Answer from the drawing. Dimensions are ordinates in mm from the lowest x, y and z of the part. A direction names the side the tool comes from. Coordinates: 2 decimals unless noted, no trailing zeros. Write each loop counter-clockwise with the first axis right and the second up, starting at its lowest first coordinate (ties: lowest second). Pieces come first, ordered by that corner, then holes. Notation, with made-up numbers: (11.5, 85.5) -> (37.5, 85.5) arc R20 ccw to (37.5, 106.5) -> close; hole circle Ø8 at (-27, -13). An arc over 180 degrees is marked (long way). Use CSV: the item, a comma, the result in double quotes.
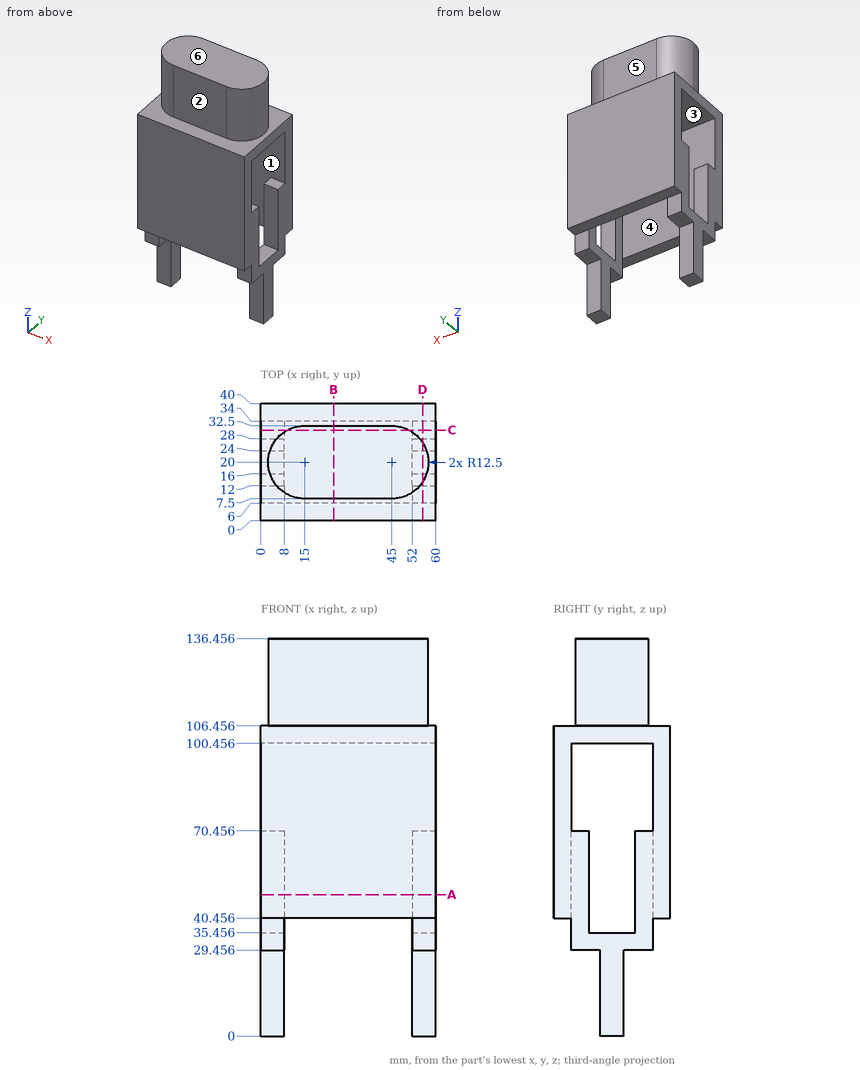
1. For a pull along Z with two mould halves and no side action, classify the marked faces 4, 5 and 6 as pulls with the +Z half, pulls with the -Z half, needs draft (parallel to the pull), parting line crosses it, or undercut.
Solutions:
face 4,"undercut"
face 5,"needs draft"
face 6,"pulls with the +Z half"
2. A cutting plane is placed at B-B (x = 25). Give the vertices of the cut face in (y, z).
Solutions:
outline,"(0, 40.46) -> (6, 40.46) -> (6, 100.46) -> (34, 100.46) -> (34, 40.46) -> (40, 40.46) -> (40, 106.46) -> (32.5, 106.46) -> (32.5, 136.46) -> (7.5, 136.46) -> (7.5, 106.46) -> (0, 106.46) -> close"
3. A cutting plane is placed at A-A (z = 48.5). Give the vertices of the cut face in (x, y).
Solutions:
outline,"(0, 0) -> (60, 0) -> (60, 12) -> (52, 12) -> (52, 6) -> (8, 6) -> (8, 12) -> (0, 12) -> close; (0, 28) -> (8, 28) -> (8, 34) -> (52, 34) -> (52, 28) -> (60, 28) -> (60, 40) -> (0, 40) -> close"
4. Find the intervals of material crossed by line 1 along Y through (x, z) = (25, 81); line 2 along X through (y, z) = (20, 9.5); line 3 along Z through (x, y) = (56.5, 18.5), in increasing order.
Solutions:
line 1,"y = 0 to 6, 34 to 40"
line 2,"x = 0 to 8, 52 to 60"
line 3,"z = 0 to 35.46, 100.46 to 136.46"
5. Each of these flat-tipped pins is pushed along its axis until it touches: pin 1 Ø9 at (x, z) = (54.5, 14) entering from +Y; pin 2 Ø2.5 at (x, z) = (4, 33.5) entering from +Y; pin 3 Ø9 at (x, y) = (5, 29) entering from -Z. Where does it stop, or does it pass through?
Solutions:
pin 1,"stops at y = 24"
pin 2,"stops at y = 34"
pin 3,"stops at z = 29.46"
6. A cutting plane is placed at C-C (y = 31). Give the vertices of the cut face in (x, z), and give its area (3 significant figures).
Solutions:
outline,"(0, 29.46) -> (8, 29.46) -> (8, 70.46) -> (0, 70.46) -> close; (0, 100.46) -> (60, 100.46) -> (60, 106.46) -> (50.94, 106.46) -> (50.94, 136.46) -> (9.06, 136.46) -> (9.06, 106.46) -> (0, 106.46) -> close; (52, 29.46) -> (60, 29.46) -> (60, 70.46) -> (52, 70.46) -> close"
area,"2,270 mm^2"
7. A cutting plane is placed at D-D (x = 55.5). Give the vertices of the cut face in (y, z).
Solutions:
outline,"(0, 40.46) -> (6, 40.46) -> (6, 29.46) -> (16, 29.46) -> (16, 0) -> (24, 0) -> (24, 29.46) -> (34, 29.46) -> (34, 40.46) -> (40, 40.46) -> (40, 106.46) -> (26.78, 106.46) -> (26.78, 136.46) -> (13.22, 136.46) -> (13.22, 106.46) -> (0, 106.46) -> close; hole (6, 70.46) -> (12, 70.46) -> (12, 35.46) -> (28, 35.46) -> (28, 70.46) -> (34, 70.46) -> (34, 100.46) -> (6, 100.46) -> close"
8. A tool of negligible diameter and unlimited length cuts with its end or side. For the marked faces 1, 2 and 3, from which of +Z, -Z, +X, -X, +Y, -Y can it reach the whole face along a straight path? Write none if from no direction.
Solutions:
face 1,"none"
face 2,"+Z, +X, -X, -Y"
face 3,"+X, -X"
